from build123d import *

# Parameters (mm, degrees)
SKETCH_1_R          = 11
EXTRUDE_1_DEPTH     = 5
SKETCH_2_R          = 4
EXTRUDE_2_DEPTH     = 3.9
SKETCH_3_R          = 1.8
CUT_EXTRUDE_1_DEPTH = 6
SKETCH_4_R          = 2
CUT_EXTRUDE_2_DEPTH = 9.9
SKETCH_6_R          = 1.25
CUT_EXTRUDE_3_DEPTH = 13


with BuildPart() as part:
    # 스케치1 → 보스-돌출1 (new body)
    with BuildSketch(Plane(origin=(0, 0, 0), x_dir=(1, 0, 0), z_dir=(0, 1, 0))):
        Circle(SKETCH_1_R)
    extrude(amount=EXTRUDE_1_DEPTH)

    # 스케치2 → 보스-돌출2 (add)
    with BuildSketch(Plane(origin=(0, 5, 0), x_dir=(1, 0, 0), z_dir=(0, 1, 0))):
        Circle(SKETCH_2_R)
    extrude(amount=EXTRUDE_2_DEPTH)

    # 스케치3 → 컷-돌출1 (cut, through all)
    with BuildSketch(Plane(origin=(0, 5, 0), x_dir=(1, 0, 0), z_dir=(0, 1, 0))):
        with Locations((5.656854249, 5.656854249)):
            Circle(SKETCH_3_R)
        with Locations((-5.656854249, -5.656854249)):
            Circle(SKETCH_3_R)
        with Locations((-5.656854249, 5.656854249)):
            Circle(SKETCH_3_R)
        with Locations((5.656854249, -5.656854249)):
            Circle(SKETCH_3_R)
    extrude(amount=-CUT_EXTRUDE_1_DEPTH, mode=Mode.SUBTRACT)

    # 스케치4 → 컷-돌출2 (cut, through all)
    with BuildSketch(Plane(origin=(0, 8.9, 0), x_dir=(1, 0, 0), z_dir=(0, 1, 0))):
        Circle(SKETCH_4_R)
    extrude(amount=-CUT_EXTRUDE_2_DEPTH, mode=Mode.SUBTRACT)

    # 스케치6 → 컷-돌출3 (cut)
    with BuildSketch(Plane.XY):
        with Locations((0, 2.5)):
            Circle(SKETCH_6_R)
    extrude(amount=-CUT_EXTRUDE_3_DEPTH, mode=Mode.SUBTRACT)


solid = part.part
Input: part model. Units: mm. Frame: model coordinates. A direction names the side the tool comes from. Round coordinates to 2 decimals unless told otherwise and drop trailing zeros. Order: outer loops, then holes, each group sorted by start corner. A loop starts at its lowest first (then second) coordinate and runs counter-clockwise, first axis right, second up.
1. Mould query, pull axis Z, two halves, no side actions, for faces 4 (the face through (-2, 8.9, 1)), 5 (the face through (7.32, 2.54, -4.97)), 6 (the face through (-2.38, 2.46, 10.74)). Classes: released by +Z, released by -Z, zero draft, split by the parting line, or undercut.
The answers:
face 4: zero draft
face 5: undercut
face 6: split by the parting line
2. Cut plane A-A, the plane x = 0. Output: boundary loops of the cut face in (y, z).
The answers:
outline: (0, -11) - (1.25, -11) - (1.25, -2) - (0, -2) - close; (0, 2) - (8.9, 2) - (8.9, 4) - (5, 4) - (5, 11) - (0, 11) - close; (3.75, -11) - (5, -11) - (5, -4) - (8.9, -4) - (8.9, -2) - (3.75, -2) - close
3. Cut plane D-D, the plane y = 5.75. Output: boundary loops of the cut face in (x, z), then the cut area to 3 significant figures.
The answers:
outline: circle Ø8 at (0, 0); hole circle Ø4 at (0, 0)
area: 37.7 mm2
4. Set-up query: faces 1 (the face through (-0.16, 3.74, -6.22)), 2 (the face through (5, 5, 0)), 3 (the face through (7.32, 2.54, 6.35)). Return all of +Z, -Z, +X, -X, +Y, -Y with unobstructed straight access to the full face (end or side cutting, diameter ignored); none if empty.
The answers:
face 1: -Z
face 2: +Y
face 3: +Y, -Y
5. Material intervals for line 1 (Z direction, x = 0, y = 6.25); line 2 (X direction, y = 2.5, z = -6.5); line 3 (X direction, y = 0.5, z = 7.25), sorted ascending.
The answers:
line 1: z = -4 to -2, 2 to 4
line 2: x = -8.87 to -7.25, -4.07 to -1.25, 1.25 to 4.07, 7.25 to 8.87
line 3: x = -8.27 to -6.49, -4.82 to 4.82, 6.49 to 8.27
6. Cut plane B-B, the plane z = 0. Output: boundary loops of the cut face in (x, y), then the cut area to 3 significant figures.
The answers:
outline: (-11, 0) - (-2, 0) - (-2, 8.9) - (-4, 8.9) - (-4, 5) - (-11, 5) - close; (2, 0) - (11, 0) - (11, 5) - (4, 5) - (4, 8.9) - (2, 8.9) - close
area: 106 mm2
7. Pin query (flat end, axial travel): P1, Ø12, axis at x = -4, z = 3.5, coming from the -Y side; P2, Ø2, axis at x = -6, z = 6.5, coming from the +Y side; P3, Ø1, axis at x = 6.5, y = 5, coming from the +Z side; P4, Ø2, axis at x = -5.66, z = -5.66, coming from the -Y side. Return the tip coordinate at first contact, or that it passes through.
The answers:
P1: stops at y = 0
P2: stops at y = 5
P3: stops at z = 9.22
P4: passes through
8. Cut plane C-C, the plane y = 2.5. Output: boundary loops of the cut face in (x, z).
The answers:
outline: (-1.25, -10.93) - (-1.25, -1.56) arc R2 cw (long way) to (1.25, -1.56) - (1.25, -10.93) arc R11 ccw (long way) to start; hole circle Ø3.6 at (-5.66, -5.66); hole circle Ø3.6 at (-5.66, 5.66); hole circle Ø3.6 at (5.66, -5.66); hole circle Ø3.6 at (5.66, 5.66)
